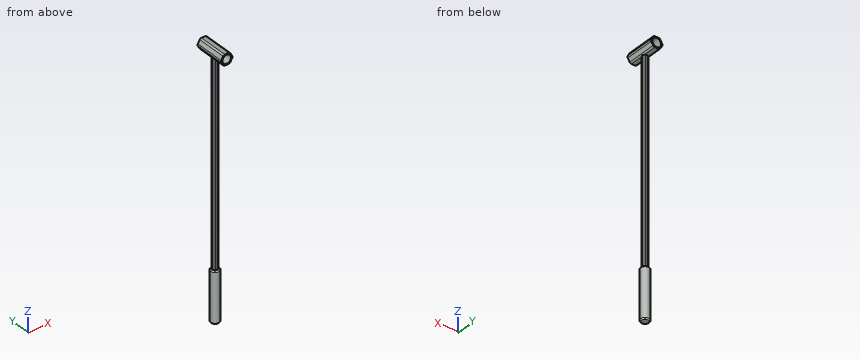
from build123d import *

# Parameters (mm, degrees)
F0_R         = 4.25
F1_DEPTH     = 30
F3_DEPTH     = 200
F4_R         = 4.25
F5_DEPTH     = 50
F6_T1_DEPTH  = 35.7735026919
F6_T6_DEPTH  = 35.7735026919
F6_T12_DEPTH = 35.7735026919
F6_T18_DEPTH = 35.7735026919
F6_T24_DEPTH = 35.7735026919
F6_T30_DEPTH = 35.7735026919
F6_T36_DEPTH = 35.7735026919
F7_R         = 1
F8_R         = 1


# Not quite as in the source:
# - a fillet or chamfer that OpenCascade refuses, or shapes differently, is made with other operations: its cross-section is extruded or revolved along the edge and cut away or added


with BuildPart() as f1:
    # F0 (on Front) → F1 (new body)
    with BuildSketch(Plane.XZ):
        Polygon((3.0310889132, 5.25), (-3.0310889132, 5.25), (-6.0621778265, 0), (-3.0310889132, -5.25), (3.0310889132, -5.25), (6.0621778265, 0), align=None)
        Circle(F0_R, mode=Mode.SUBTRACT)
    extrude(amount=F1_DEPTH)

    # F2 (on face) → F3 (join)
    with BuildSketch(Plane(origin=(0, 0, -5.25), x_dir=(1, 0, 0), z_dir=(0, 0, -1))):
        Polygon((-1.443375673, 12.5), (0, 12.5), (1.443375673, 12.5), (2.8867513459, 15), (1.443375673, 17.5), (-1.443375673, 17.5), (-2.8867513459, 15), align=None)
    extrude(amount=F3_DEPTH)

    # F4 (on face) → F5 (join)
    with BuildSketch(Plane(origin=(0, 0, -205.25), x_dir=(1, 0, 0), z_dir=(0, 0, -1))):
        with Locations((0, 15)):
            Circle(F4_R)
        Polygon((-1.443375673, 12.5), (-2.8867513459, 15), (-1.443375673, 17.5), (1.443375673, 17.5), (2.8867513459, 15), (1.443375673, 12.5), align=None, mode=Mode.SUBTRACT)
        Polygon((-1.443375673, 17.5), (-2.8867513459, 15), (-1.443375673, 12.5), (1.443375673, 12.5), (2.8867513459, 15), (1.443375673, 17.5), align=None)
    extrude(amount=F5_DEPTH)

    # F6: fillet of radius 2 on 6 edges, made by hand

    # F6_s2 → F6_t1 (cut)
    with BuildSketch(Plane.XZ.offset(-2.8867513459)):
        with BuildLine():
            ThreePointArc((5.4848275573, -1), (5.7527767497, 0), (5.4848275573, 1))
            Line((5.4848275573, 1), (6.0621778265, 0))
            Line((6.0621778265, 0), (5.4848275573, -1))
        make_face()
        with BuildLine():
            ThreePointArc((1.8763883749, 5.25), (2.8763883749, 4.9820508076), (3.6084391824, 4.25))
            Line((3.6084391824, 4.25), (3.0310889132, 5.25))
            Line((3.0310889132, 5.25), (1.8763883749, 5.25))
        make_face()
        with BuildLine():
            ThreePointArc((-3.6084391824, 4.25), (-2.8763883749, 4.9820508076), (-1.8763883749, 5.25))
            Line((-1.8763883749, 5.25), (-3.0310889132, 5.25))
            Line((-3.0310889132, 5.25), (-3.6084391824, 4.25))
        make_face()
        with BuildLine():
            ThreePointArc((-5.4848275573, -1), (-5.7527767497, 0), (-5.4848275573, 1))
            Line((-5.4848275573, 1), (-6.0621778265, 0))
            Line((-6.0621778265, 0), (-5.4848275573, -1))
        make_face()
    extrude(amount=F6_T1_DEPTH, mode=Mode.SUBTRACT)


with BuildPart() as f6_tool4:
    # F6_s5 → F6_t6 (new body)
    with BuildSketch(Plane.XZ.offset(-2.8867513459)):
        with BuildLine():
            ThreePointArc((1.8763883749, -5.25), (2.8763883749, -4.9820508076), (3.6084391824, -4.25))
            Line((3.6084391824, -4.25), (3.0310889132, -5.25))
            Line((3.0310889132, -5.25), (1.8763883749, -5.25))
        make_face()
    extrude(amount=F6_T6_DEPTH)

    split(bisect_by=Plane(origin=(-4.3301270189, -2.5, 0), x_dir=(0, 0, 1), z_dir=(0.8660254038, 0.5, 0)), keep=Keep.TOP)

    split(bisect_by=Plane(origin=(8.6602540378, -5, 0), x_dir=(0, 0, 1), z_dir=(-0.8660254038, 0.5, 0)), keep=Keep.TOP)


with BuildPart() as f1_1:
    add(f1.part)

    # F6_t3: cut F6_tool4
    add(f6_tool4.part, mode=Mode.SUBTRACT)


with BuildPart() as f6_tool10:
    # F6_s11 → F6_t12 (new body)
    with BuildSketch(Plane.XZ.offset(-2.8867513459)):
        with BuildLine():
            ThreePointArc((1.8763883749, -5.25), (2.8763883749, -4.9820508076), (3.6084391824, -4.25))
            Line((3.6084391824, -4.25), (3.0310889132, -5.25))
            Line((3.0310889132, -5.25), (1.8763883749, -5.25))
        make_face()
    extrude(amount=F6_T12_DEPTH)

    split(bisect_by=Plane(origin=(-4.3301270189, -2.5, 0), x_dir=(0, 0, 1), z_dir=(0.8660254038, 0.5, 0)), keep=Keep.TOP)

    split(bisect_by=Plane(origin=(8.6602540378, -5, 0), x_dir=(0, 0, 1), z_dir=(0.8660254038, -0.5, 0)), keep=Keep.TOP)


with BuildPart() as f1_2:
    add(f1_1.part)

    # F6_t9: cut F6_tool10
    add(f6_tool10.part, mode=Mode.SUBTRACT)


with BuildPart() as f6_tool16:
    # F6_s17 → F6_t18 (new body)
    with BuildSketch(Plane.XZ.offset(-2.8867513459)):
        with BuildLine():
            ThreePointArc((1.8763883749, -5.25), (2.8763883749, -4.9820508076), (3.6084391824, -4.25))
            Line((3.6084391824, -4.25), (3.0310889132, -5.25))
            Line((3.0310889132, -5.25), (1.8763883749, -5.25))
        make_face()
    extrude(amount=F6_T18_DEPTH)

    split(bisect_by=Plane(origin=(-4.3301270189, -2.5, 0), x_dir=(0, 0, 1), z_dir=(-0.8660254038, -0.5, 0)), keep=Keep.TOP)

    split(bisect_by=Plane(origin=(8.6602540378, -5, 0), x_dir=(0, 0, 1), z_dir=(0.8660254038, -0.5, 0)), keep=Keep.TOP)


with BuildPart() as f1_3:
    add(f1_2.part)

    # F6_t15: cut F6_tool16
    add(f6_tool16.part, mode=Mode.SUBTRACT)


with BuildPart() as f6_tool22:
    # F6_s23 → F6_t24 (new body)
    with BuildSketch(Plane.XZ.offset(-2.8867513459)):
        with BuildLine():
            ThreePointArc((-1.8763883749, -5.25), (-2.8763883749, -4.9820508076), (-3.6084391824, -4.25))
            Line((-3.6084391824, -4.25), (-3.0310889132, -5.25))
            Line((-3.0310889132, -5.25), (-1.8763883749, -5.25))
        make_face()
    extrude(amount=F6_T24_DEPTH)

    split(bisect_by=Plane(origin=(-8.6602540378, -5, 0), x_dir=(0, 0, 1), z_dir=(0.8660254038, 0.5, 0)), keep=Keep.TOP)

    split(bisect_by=Plane(origin=(4.3301270189, -2.5, 0), x_dir=(0, 0, 1), z_dir=(-0.8660254038, 0.5, 0)), keep=Keep.TOP)


with BuildPart() as f1_4:
    add(f1_3.part)

    # F6_t21: cut F6_tool22
    add(f6_tool22.part, mode=Mode.SUBTRACT)


with BuildPart() as f6_tool28:
    # F6_s29 → F6_t30 (new body)
    with BuildSketch(Plane.XZ.offset(-2.8867513459)):
        with BuildLine():
            ThreePointArc((-1.8763883749, -5.25), (-2.8763883749, -4.9820508076), (-3.6084391824, -4.25))
            Line((-3.6084391824, -4.25), (-3.0310889132, -5.25))
            Line((-3.0310889132, -5.25), (-1.8763883749, -5.25))
        make_face()
    extrude(amount=F6_T30_DEPTH)

    split(bisect_by=Plane(origin=(-8.6602540378, -5, 0), x_dir=(0, 0, 1), z_dir=(-0.8660254038, -0.5, 0)), keep=Keep.TOP)

    split(bisect_by=Plane(origin=(4.3301270189, -2.5, 0), x_dir=(0, 0, 1), z_dir=(-0.8660254038, 0.5, 0)), keep=Keep.TOP)


with BuildPart() as f1_5:
    add(f1_4.part)

    # F6_t27: cut F6_tool28
    add(f6_tool28.part, mode=Mode.SUBTRACT)


with BuildPart() as f6_tool34:
    # F6_s35 → F6_t36 (new body)
    with BuildSketch(Plane.XZ.offset(-2.8867513459)):
        with BuildLine():
            ThreePointArc((-1.8763883749, -5.25), (-2.8763883749, -4.9820508076), (-3.6084391824, -4.25))
            Line((-3.6084391824, -4.25), (-3.0310889132, -5.25))
            Line((-3.0310889132, -5.25), (-1.8763883749, -5.25))
        make_face()
    extrude(amount=F6_T36_DEPTH)

    split(bisect_by=Plane(origin=(-8.6602540378, -5, 0), x_dir=(0, 0, 1), z_dir=(-0.8660254038, -0.5, 0)), keep=Keep.TOP)

    split(bisect_by=Plane(origin=(4.3301270189, -2.5, 0), x_dir=(0, 0, 1), z_dir=(0.8660254038, -0.5, 0)), keep=Keep.TOP)


with BuildPart() as f1_6:
    add(f1_5.part)

    # F6_t33: cut F6_tool34
    add(f6_tool34.part, mode=Mode.SUBTRACT)

    # F7
    f7_edges = [f1_6.edges().sort_by_distance(p)[0] for p in [
        (-1.443376, -17.5, -105.25),
        (1.443376, -17.5, -105.25),
        (-2.886751, -15, -105.113013),
        (-1.443376, -12.5, -105.25),
        (2.886751, -15, -105.113013),
        (1.443376, -12.5, -105.25),
    ]]
    fillet(f7_edges, radius=F7_R)

    # F8
    f8_edges = [f1_6.edges().sort_by_distance(p)[0] for p in [
        (-4.25, -15, -255.25),
        (-4.25, -15, -205.25),
    ]]
    fillet(f8_edges, radius=F8_R)


solid = f1_6.part
Could you check a few things on this model? Use its own coordinates, in mm. Coordinates: 2 decimals unless noted, no trailing zeros. Loops run counter-clockwise (first coordinate to the right, second up) from the corner with the lowest first, then second, coordinate; pieces in that order, holes last.
1. I need wall thicknesses on L1, parallel to Z at x = -2.25, y = -20; L2, parallel to Z at x = 0.5, y = -0.5; L3, parallel to Y at x = 1, z = -197. Which ranges of each line are inside material? Lowest first, please.
2. For P1, Ø1.9, axis at x = 1, y = -23, coming from the -Z side; P2, Ø6, axis at x = -3, z = -161.5, coming from the -Y side; P3, Ø0.5, axis at x = 0, z = -147, coming from the +Y side, each with a flat end and sliding along its axis, tell me the tip position at first contact or that it passes through.
3. Imagine slicing it at A-A (y = -5.5). Please give me the cut outline in (x, z), and give its area (3 significant figures).
4. Imagine slicing it at B-B (z = -56). Please give me the cut outline in (x, y).
Computed values:
1. L1: z = -5.21 to -3.61, 3.61 to 5.21
1. L2: z = -5.25 to -4.22, 4.22 to 5.25
1. L3: y = -17.49 to -12.51
2. P1: stops at z = -5.25
2. P2: stops at y = -17.5
2. P3: stops at y = -12.5
3. outline: (-5.48, -1) - (-3.61, -4.25) arc R2 ccw to (-1.88, -5.25) - (1.88, -5.25) arc R2 ccw to (3.61, -4.25) - (5.48, -1) arc R2 ccw to (5.48, 1) - (3.61, 4.25) arc R2 ccw to (1.88, 5.25) - (-1.88, 5.25) arc R2 ccw to (-3.61, 4.25) - (-5.48, 1) arc R2 ccw to start; hole circle Ø8.5 at (0, 0)
3. area: 37.4 mm2
4. outline: (-2.6, -15.5) - (-1.73, -17) arc R1 ccw to (-0.87, -17.5) - (0.87, -17.5) arc R1 ccw to (1.73, -17) - (2.6, -15.5) arc R1 ccw to (2.6, -14.5) - (1.73, -13) arc R1 ccw to (0.87, -12.5) - (-0.87, -12.5) arc R1 ccw to (-1.73, -13) - (-2.6, -14.5) arc R1 ccw to start
